from build123d import *

# Parameters (mm, degrees)
BOSS_EXTRUDE1_DEPTH         = 2.54
F_11_0_191_DIAMETER_HOLE2_D = 4.8514
F_11_0_191_DIAMETER_HOLE3_D = 4.8514
SKETCH17_W                  = 6.35
SKETCH17_H                  = 50.8
SKETCH17_W_2                = 50.8
SKETCH17_H_2                = 6.35
SKETCH17_H_3                = 25.4
CUT_EXTRUDE12_DEPTH         = 304.883162745
MIRROR1_OUTLINE_W           = 6.35
MIRROR1_OUTLINE_H           = 50.8
MIRROR1_OUTLINE_R           = 2.4257
MIRROR1_OUTLINE_W_2         = 50.8
MIRROR1_OUTLINE_H_2         = 6.35
MIRROR1_DEPTH               = 2.54


# Read off the part's stored shape, not the designer's step: Mirror1
with BuildPart() as part:
    # Sketch1 → Boss-Extrude1 (new body)
    with BuildSketch(Plane(origin=(0, 0, 0), x_dir=(1, 0, 0), z_dir=(0, 1, 0))):
        Polygon((0, 63.5), (-273.05, 63.5), (-273.05, -63.5), (-273.05, -133.35), (273.05, -133.35), (273.05, -63.5), (273.05, 63.5), align=None)
    extrude(amount=BOSS_EXTRUDE1_DEPTH)

    # 11 _0.191_ Diameter Hole2 (through all)
    with Locations(Plane(origin=(0, 2.54, 0), x_dir=(1, 0, 0), z_dir=(0, 1, 0))):
        with Locations((-119.126, -56.127777467), (-38.862, -56.127777467), (38.862, -56.127777467), (119.126, -56.127777467)):
            Hole(F_11_0_191_DIAMETER_HOLE2_D / 2)

    # 11 _0.191_ Diameter Hole3 (through all)
    with Locations(Plane(origin=(0, 2.54, 0), x_dir=(1, 0, 0), z_dir=(0, 1, 0))):
        with Locations((119.126, 63.5), (38.862, 63.5)):
            Hole(F_11_0_191_DIAMETER_HOLE3_D / 2)

    # Sketch17 → Cut-Extrude12 (cut, through all)
    with BuildSketch(Plane(origin=(0, 2.54, 0), x_dir=(1, 0, 0), z_dir=(0, 1, 0))):
        with Locations((-263.525, -57.15)):
            Rectangle(SKETCH17_W, SKETCH17_H)
        with Locations((-190.5, -123.825)):
            Rectangle(SKETCH17_W_2, SKETCH17_H_2)
        with Locations((190.5, -123.825)):
            Rectangle(SKETCH17_W_2, SKETCH17_H_2)
        with Locations((263.525, -57.15)):
            Rectangle(SKETCH17_W, SKETCH17_H)
        with Locations((0, -123.825)):
            Rectangle(SKETCH17_W_2, SKETCH17_H_2)
        with Locations((-263.525, 50.8)):
            Rectangle(SKETCH17_W, SKETCH17_H_3)
        with Locations((263.525, 50.8)):
            Rectangle(SKETCH17_W, SKETCH17_H_3)
    extrude(amount=-CUT_EXTRUDE12_DEPTH, mode=Mode.SUBTRACT)

    # Mirror1 outline → Mirror1 (add)
    with BuildSketch(Plane(origin=(0, 0, 0), x_dir=(1, 0, 0), z_dir=(0, 1, 0))):
        with BuildLine():
            Line((273.05, 63.5), (273.05, 260.35))
            Line((273.05, 260.35), (-273.05, 260.35))
            Line((-273.05, 260.35), (-273.05, 63.5))
            Line((-273.05, 63.5), (-266.7, 63.5))
            Line((-266.7, 63.5), (-266.7, 88.9))
            Line((-266.7, 88.9), (-260.35, 88.9))
            Line((-260.35, 88.9), (-260.35, 63.5))
            Line((-260.35, 63.5), (36.4363, 63.5))
            ThreePointArc((36.4363, 63.5), (38.862, 65.9257), (41.2877, 63.5))
            Line((41.2877, 63.5), (116.7003, 63.5))
            ThreePointArc((116.7003, 63.5), (119.126, 65.9257), (121.5517, 63.5))
            Line((121.5517, 63.5), (260.35, 63.5))
            Line((260.35, 63.5), (260.35, 88.9))
            Line((260.35, 88.9), (266.7, 88.9))
            Line((266.7, 88.9), (266.7, 63.5))
            Line((266.7, 63.5), (273.05, 63.5))
        make_face()
        with Locations((-263.525, 184.15)):
            Rectangle(MIRROR1_OUTLINE_W, MIRROR1_OUTLINE_H, mode=Mode.SUBTRACT)
        with Locations((-119.126, 183.127777467)):
            Circle(MIRROR1_OUTLINE_R, mode=Mode.SUBTRACT)
        with Locations((-38.862, 183.127777467)):
            Circle(MIRROR1_OUTLINE_R, mode=Mode.SUBTRACT)
        with Locations((-190.5, 250.825)):
            Rectangle(MIRROR1_OUTLINE_W_2, MIRROR1_OUTLINE_H_2, mode=Mode.SUBTRACT)
        with Locations((38.862, 183.127777467)):
            Circle(MIRROR1_OUTLINE_R, mode=Mode.SUBTRACT)
        with Locations((119.126, 183.127777467)):
            Circle(MIRROR1_OUTLINE_R, mode=Mode.SUBTRACT)
        with Locations((263.525, 184.15)):
            Rectangle(MIRROR1_OUTLINE_W, MIRROR1_OUTLINE_H, mode=Mode.SUBTRACT)
        with Locations((0, 250.825)):
            Rectangle(MIRROR1_OUTLINE_W_2, MIRROR1_OUTLINE_H_2, mode=Mode.SUBTRACT)
        with Locations((190.5, 250.825)):
            Rectangle(MIRROR1_OUTLINE_W_2, MIRROR1_OUTLINE_H_2, mode=Mode.SUBTRACT)
    extrude(amount=MIRROR1_DEPTH)


solid = part.part
Check sheet for the modelled part. Datum: model origin and axes. Units: mm. Give positions to 0.01 mm unless a question says otherwise; leave off trailing zeros. Write each loop counter-clockwise with the first axis right and the second up, starting at its lowest first coordinate (ties: lowest second). Pieces come first, ordered by that corner, then holes. Notation, with made-up numbers: (-9, 65) -> (40, 65) arc R13 ccw to (40, 89) -> close; hole circle Ø3 at (43, 70). An arc over 180 degrees is marked (long way). One line per item, written item: value. Start each with the question number.
Item 1: Material ranges on probe 1 along Z at (x, y) = (118.5, 2); probe 2 along X at (y, z) = (0.9, 42.5); probe 3 along Z at (x, y) = (10.5, 0.7), recorded low to high. Write a range as from..to.
Item 2: Section check B-B on y = 0.4. State how many separate pieces and enclosed holes the cut face has, then the cut area to 3 significant figures.
Item 3: Section check A-A on z = -168. Record the cut outline in (x, y).
Results list:
1. probe 1: -260.35..-185.47, -180.78..-65.84, -61.16..53.78, 58.47..133.35
1. probe 2: -273.05..-266.7, -260.35..260.35, 266.7..273.05
1. probe 3: -260.35..-254, -247.65..120.65, 127..133.35
2. separate pieces: 1
2. enclosed holes: 22
2. area: 211,000 mm²
3. outline: (-273.05, 0) -> (-266.7, 0) -> (-266.7, 2.54) -> (-273.05, 2.54) -> close; (-260.35, 0) -> (260.35, 0) -> (260.35, 2.54) -> (-260.35, 2.54) -> close; (266.7, 0) -> (273.05, 0) -> (273.05, 2.54) -> (266.7, 2.54) -> close
